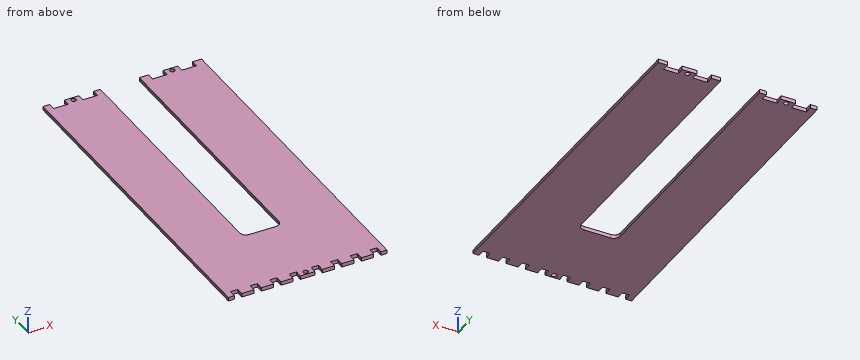
from build123d import *

# Parameters (mm, degrees)
ESQUISSE1_W             = 130
ESQUISSE1_H             = 282
BOSS_EXTRU_1_DEPTH      = 3
ESQUISSE2_W             = 32
ESQUISSE2_H             = 217
ENL_V_MAT_EXTRU_1_DEPTH = 3
CONG_1_R                = 5
ESQUISSE3_R             = 2
ESQUISSE3_W             = 12
ESQUISSE3_H             = 6
ESQUISSE3_W_2           = 6
ENL_V_MAT_EXTRU_2_DEPTH = 3


with BuildPart() as part:
    # Esquisse1 → Boss.-Extru.1 (new body)
    with BuildSketch(Plane.XY):
        with Locations((18.458602023, -91.280290456)):
            Rectangle(ESQUISSE1_W, ESQUISSE1_H)
    extrude(amount=BOSS_EXTRU_1_DEPTH)

    # Esquisse2 → Enlèv. mat.-Extru.1 (cut)
    with BuildSketch(Plane.XY.offset(3)):
        with Locations((16.458602023, -58.780290456)):
            Rectangle(ESQUISSE2_W, ESQUISSE2_H)
    extrude(amount=-ENL_V_MAT_EXTRU_1_DEPTH, mode=Mode.SUBTRACT)

    # Congé1
    cong_1_edges = [part.edges().sort_by_distance(p)[0] for p in [
        (32.458602023, -167.280290456, 1.5),
        (0.458602023, -167.280290456, 1.5),
    ]]
    fillet(cong_1_edges, radius=CONG_1_R)

    # Esquisse3 → Enlèv. mat.-Extru.2 (cut)
    with BuildSketch(Plane.XY.offset(3)):
        with Locations((-23.041397977, 46.719709544)):
            Circle(ESQUISSE3_R)
        with Locations((57.958602023, 46.719709544)):
            Circle(ESQUISSE3_R)
        with Locations((18.458602023, -229.280290456)):
            Circle(ESQUISSE3_R)
        with Locations((-35.041397977, 46.719709544)):
            Rectangle(ESQUISSE3_W, ESQUISSE3_H)
        with Locations((-11.041397977, 46.719709544)):
            Rectangle(ESQUISSE3_W, ESQUISSE3_H)
        with Locations((45.958602023, 46.719709544)):
            Rectangle(ESQUISSE3_W, ESQUISSE3_H)
        with Locations((69.958602023, 46.719709544)):
            Rectangle(ESQUISSE3_W, ESQUISSE3_H)
        with Locations((9.458602023, -229.280290456)):
            Rectangle(ESQUISSE3_W_2, ESQUISSE3_H)
        with Locations((-6.541397977, -229.280290456)):
            Rectangle(ESQUISSE3_W_2, ESQUISSE3_H)
        with Locations((-38.541397977, -229.280290456)):
            Rectangle(ESQUISSE3_W_2, ESQUISSE3_H)
        with Locations((27.458602023, -229.280290456)):
            Rectangle(ESQUISSE3_W_2, ESQUISSE3_H)
        with Locations((43.458602023, -229.280290456)):
            Rectangle(ESQUISSE3_W_2, ESQUISSE3_H)
        with Locations((75.458602023, -229.280290456)):
            Rectangle(ESQUISSE3_W_2, ESQUISSE3_H)
        with Locations((-22.541397977, -229.280290456)):
            Rectangle(ESQUISSE3_W_2, ESQUISSE3_H)
        with Locations((59.458602023, -229.280290456)):
            Rectangle(ESQUISSE3_W_2, ESQUISSE3_H)
    extrude(amount=-ENL_V_MAT_EXTRU_2_DEPTH, mode=Mode.SUBTRACT)


solid = part.part
Here's how the part is built. I have some questions about the finished solid (model axes, mm). Coordinates: 2 decimals unless noted, no trailing zeros. Loops run counter-clockwise (first coordinate to the right, second up) from the corner with the lowest first, then second, coordinate; pieces in that order, holes last. Notation, with made-up numbers: (-16.75, 67.5) -> (31.25, 67.5) arc R22 cw to (31.25, 99.5) -> close; hole circle Ø4 at (42.25, -13.75). An arc over 180 degrees is marked (long way). Use one line per item in the form item = value. Start each with the question number.
(1) Please list where these lines run through material, in increasing order: line 1 along X through (y, z) = (-5, 2.5); line 2 along Y through (x, z) = (58, 1); line 3 along Y through (x, z) = (7, 1.05).
(2) Will this pin go through, and if not, where does the flat tip stop? pin 1 (1.5 mm diameter, centred on x = 74.5, z = 1, fed in from -Y).
(3) If we section it at C-C (z = 1.05): Give the number of separate pieces and of enclosed holes in the cut face, then the cut area to 3 significant figures.
(4) If we section it at B-B (x = -32): Please give me the cut outline in (y, z), then the cut area to 3 significant figures.
(5) If we section it at A-A (y = -28): Please give me the cut outline in (x, z).
Verdict:
q1.line_1 = -46.54 to 0.46, 32.46 to 83.46
q1.line_2 = -226.28 to 44.72, 48.72 to 49.72
q1.line_3 = -226.28 to -167.28
q2.pin_1 = -226.28
q3.separate_pieces = 1
q3.enclosed_holes = 3
q3.area = 29,100 mm²
q4.outline = (-232.28, 0) -> (43.72, 0) -> (43.72, 3) -> (-232.28, 3) -> close
q4.area = 828 mm²
q5.outline = (-46.54, 0) -> (0.46, 0) -> (0.46, 3) -> (-46.54, 3) -> close; (32.46, 0) -> (83.46, 0) -> (83.46, 3) -> (32.46, 3) -> close
